Design review of the part shown in the three views and the two pictorial views. Dimensions are in mm from the part's minimum x, y and z. A direction names the side the tool comes from. Give positions to 0.01 mm unless a question says otherwise; leave off trailing zeros. Write each loop counter-clockwise with the first axis right and the second up, starting at its lowest first coordinate (ties: lowest second). Pieces come first, ordered by that corner, then holes. Notation, with made-up numbers: M -28,87 L 17,87 A22 ccw 17,119 Z; hole C -11,18.25 d8. An arc over 180 degrees is marked long. Use one line per item in the form item = value. Start each with the question number.
Q1. Consider section A-A on x = 30. Write out the cut boundary in (y, z).
Q2. Clearance check with flat-ended pins moving along their axes: pin 1 Ø1 at (x, y) = (15, 15.5) entering from -Z; pin 2 Ø2 at (x, z) = (23.5, 4.5) entering from -Y; pin 3 Ø1.5 at (x, z) = (37.5, 12.5) entering from +Y; pin 4 Ø3 at (x, y) = (30, 30) entering from +Z. State where each tip first meets the part, or that it passes through.
Q3. Consider section D-D on y = 48. Write out the cut boundary in (x, z).
Q4. For probe 1 along Y at (x, z) = (30, 9.5); probe 2 along Y at (x, z) = (30, 13); probe 3 along Z at (x, y) = (40.5, 7), list the stretches that pass through material, from the lowest coordinate up. Write a range as [from, to].
Q5. Tool access review of the marked faces 1 and 2: name each direction out of +Z, -Z, +X, -X, +Y, -Y from which nothing blocks a thin tool from reaching the whole face with its end or side.
Q6. Consider section C-C on z = 12.25. Write out the cut boundary in (x, y), and give its area (3 significant figures).
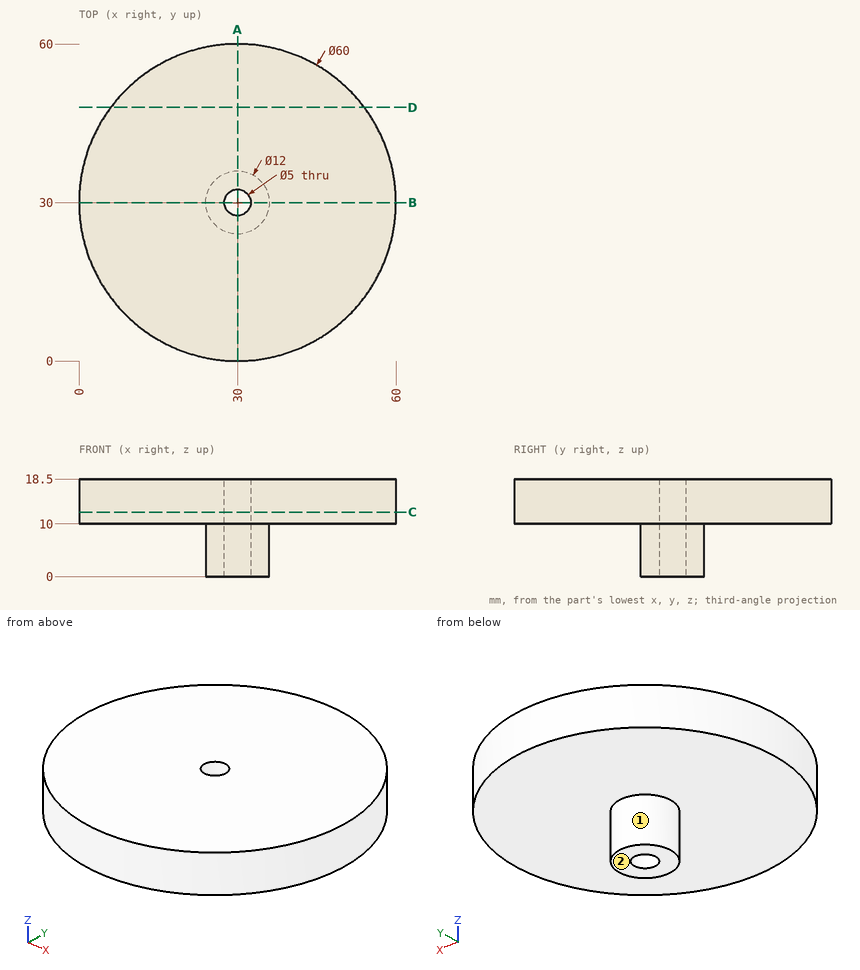
Working result:
q1.outline = M 0,10 L 24,10 L 24,0 L 27.5,0 L 27.5,18.5 L 0,18.5 Z; M 32.5,0 L 36,0 L 36,10 L 60,10 L 60,18.5 L 32.5,18.5 Z
q2.pin_1 = 10
q2.pin_2 = 27.6
q2.pin_3 = 59.23
q2.pin_4 = through
q3.outline = M 6,10 L 54,10 L 54,18.5 L 6,18.5 Z
q4.probe_1 = [24, 27.5], [32.5, 36]
q4.probe_2 = [0, 27.5], [32.5, 60]
q4.probe_3 = [10, 18.5]
q5.face_1 = -Z
q5.face_2 = -Z, +X, -X, +Y, -Y
q6.outline = C 30,30 d60; hole C 30,30 d5
q6.area = 2,810 mm²
